For this review, use the dimensioned drawing (mm, ordinates from the lowest corner) and the shaded views. Coordinates: 2 decimals unless noted, no trailing zeros. Loops run counter-clockwise (first coordinate to the right, second up) from the corner with the lowest first, then second, coordinate; pieces in that order, holes last. Notation, with made-up numbers: (25, 28) - (67, 28) arc R27 ccw to (67, 51) - close; hole circle Ø8 at (9, 70). An arc over 180 degrees is marked (long way). Use one line per item in the form item = value. Start each with the question number.
(1) Add section B-B (x = 105). State the section outline as (y, z) points.
(2) Add section D-D (z = 67.31). State the section outline as (x, y) points, plus the area to 3 significant figures.
(3) Add section C-C (y = 3). Count the separate pieces of the cut face and the enclosed holes in it, plus the area to 3 significant figures.
(4) Add section A-A (z = 16.5). State the section outline as (x, y) points.
(5) For L1, parallel to Z at x = 89.5, y = 10.75; L2, parallel to X at y = 4.25, z = 70 (3 decimals); L3, parallel to Z at x = 16, y = 10.25, list the stretches that pass through material, from the lowest coordinate up.
(6) The part is to be moulded in two halves that separate along X. For the marked faces 1, 2, 3 and 4, say which applies: pulls with the +X half, pulls with the -X half, needs draft (parallel to the pull), parting line crosses it, or undercut.
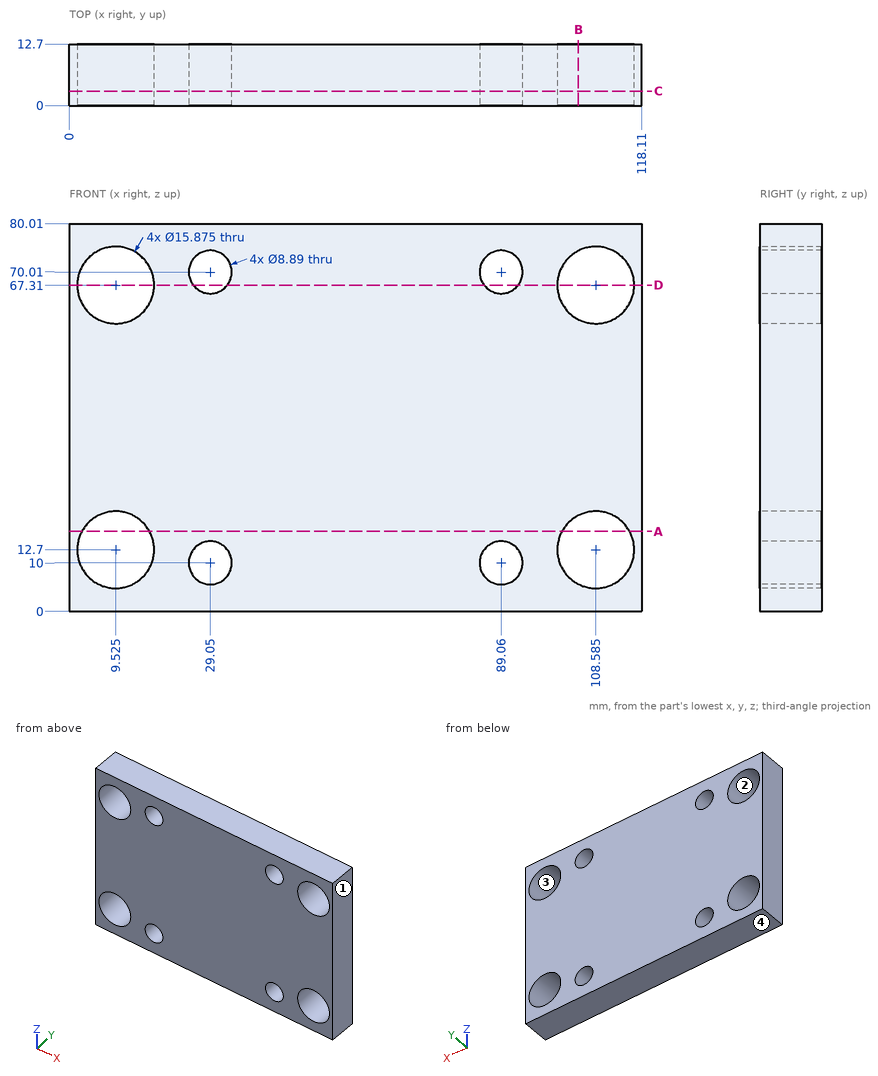
Computed values:
q1.outline = (0, 0) - (12.7, 0) - (12.7, 5.62) - (0, 5.62) - close; (0, 19.78) - (12.7, 19.78) - (12.7, 60.23) - (0, 60.23) - close; (0, 74.39) - (12.7, 74.39) - (12.7, 80.01) - (0, 80.01) - close
q2.outline = (0, 0) - (1.59, 0) - (1.59, 12.7) - (0, 12.7) - close; (17.46, 0) - (25.52, 0) - (25.52, 12.7) - (17.46, 12.7) - close; (32.58, 0) - (85.53, 0) - (85.53, 12.7) - (32.58, 12.7) - close; (92.59, 0) - (100.65, 0) - (100.65, 12.7) - (92.59, 12.7) - close; (116.52, 0) - (118.11, 0) - (118.11, 12.7) - (116.52, 12.7) - close
q2.area = 917 mm^2
q3.separate_pieces = 1
q3.enclosed_holes = 8
q3.area = 8,410 mm^2
q4.outline = (0, 0) - (2.56, 0) - (2.56, 12.7) - (0, 12.7) - close; (16.49, 0) - (101.62, 0) - (101.62, 12.7) - (16.49, 12.7) - close; (115.55, 0) - (118.11, 0) - (118.11, 12.7) - (115.55, 12.7) - close
q5.L1 = 0 to 5.58, 14.42 to 65.59, 74.43 to 80.01
q5.L2 = 0 to 2.057, 16.993 to 24.605, 33.495 to 84.615, 93.505 to 101.117, 116.053 to 118.11
q5.L3 = 0 to 8.11, 17.29 to 62.72, 71.9 to 80.01
q6.face_1 = pulls with the +X half
q6.face_2 = undercut
q6.face_3 = undercut
q6.face_4 = needs draft
